Input: dimensioned drawing with shaded views. Units: mm. Origin: part minimum x, y, z. A direction names the side the tool comes from. Give positions to 0.01 mm unless a question says otherwise; leave off trailing zeros. Write each loop counter-clockwise with the first axis right and the second up, starting at its lowest first coordinate (ties: lowest second). Pieces come first, ordered by that corner, then holes.
Q1. Section A-A (y = 10.75). Return the cut outline in (x, z).
Q2. Mould query, pull axis Y, two halves, no side actions, for the marked faces 3, 4 and 5. Classes: +Y half, -Y half, draft (parallel to the pull), parting line (faces both ways), or undercut.
Q3. Pin query (flat end, axial travel): pin 1 Ø1 at (x, z) = (5.5, 2) entering from -Y; pin 2 Ø3 at (x, y) = (2.286, 8.509) entering from +Z. Return the tip coordinate at first contact, or that it passes through.
Q4. Section C-C (z = 2.05). State how many separate pieces and enclosed holes the cut face has, plus the area to 3 significant figures.
Q5. Line query: line 1 (Y direction, x = 11, z = 2.75) (1 decimal); line 2 (Y direction, x = 3.25, z = 3.5) (1 decimal); line 3 (X direction, y = 4, z = 2.55) (1 decimal). Output: solid intervals per line, ascending.
Q6. Reachability of the marked faces 1 and 2 from +Z, -Z, +X, -X, +Y, -Y: full face, straight path, thin tool, end or side. Return the list, or none.
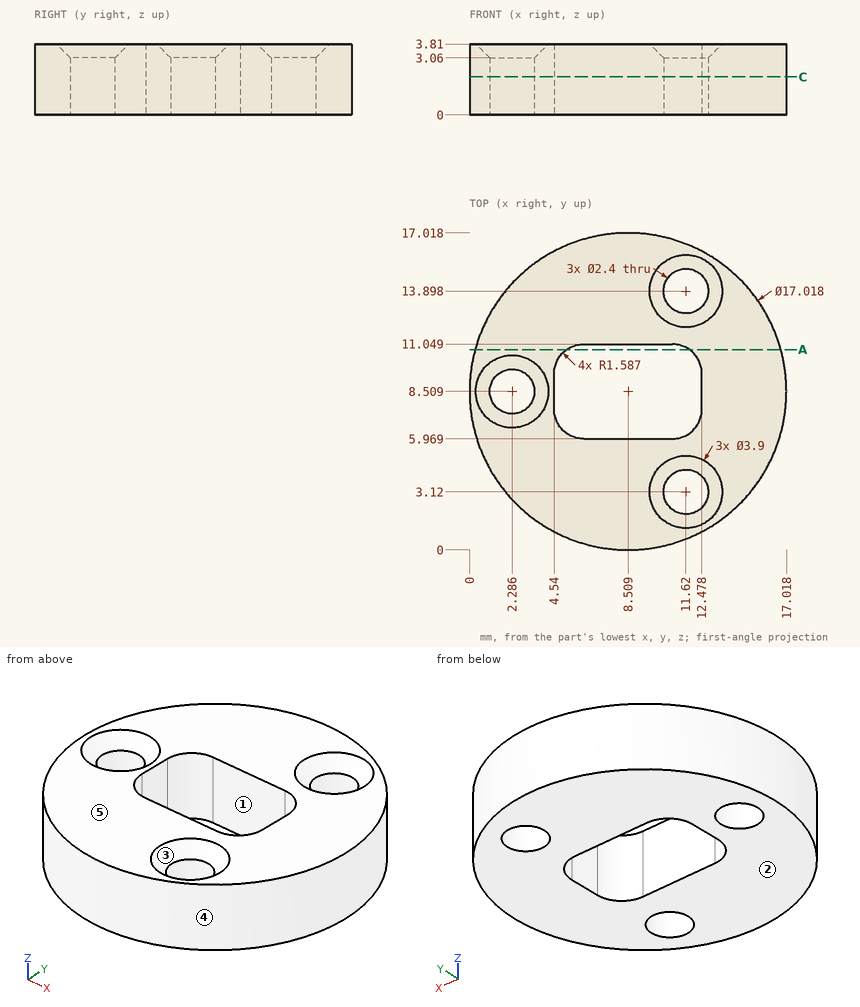
Computed:
1. outline: (0.3, 0) - (5.2, 0) - (5.2, 3.81) - (0.3, 3.81) - close; (11.82, 0) - (16.72, 0) - (16.72, 3.81) - (11.82, 3.81) - close
2. face 3: undercut
2. face 4: parting line
2. face 5: draft
3. pin 1: stops at y = 0.38
3. pin 2: stops at z = 3.36
4. separate pieces: 1
4. enclosed holes: 4
4. area: 176 mm2
5. line 1: y = 0.4 to 2.1, 4.1 to 6, 11 to 12.9, 14.9 to 16.6
5. line 2: y = 1.8 to 7.2, 9.8 to 15.2
5. line 3: x = 1.3 to 10.8, 12.4 to 15.7
6. face 1: +Z, -Z
6. face 2: -Z, +X, -X, +Y, -Y
